Verification items for the finished model (mm, model axes). Face numbers are marked on the shaded views. A direction names the side the tool comes from. Coordinates: 2 decimals unless noted, no trailing zeros. Order: outer loops, then holes, each group sorted by start corner. A loop starts at its lowest first (then second) coordinate and runs counter-clockwise, first axis right, second up. Notation, with made-up numbers: (71, -35) -> (119, -35) arc R27 cw to (119, -14) -> close; hole circle Ø5 at (-28, 37). An arc over 180 degrees is marked (long way). Write item = value, one per line. Start each with the question number.
1. Set-up check for the marked faces 5, 6, 7, 8 and 9: record each of +Z, -Z, +X, -X, +Y, -Y from which the full face is reachable in a straight line by a thin tool's end or side.
2. Release check for a two-part mould opening along X. For the marked faces 1, 2, 3 and 4 record: +X half, -X half, draft (parallel to the pull), parting line (faces both ways), or undercut.
3. Cross-section at A-A on x = -8. Record the cut outline in (y, z), plus the area to 3 significant figures.
4. Cross-section at C-C on x = 0.5. Record the cut outline in (y, z), plus the area to 3 significant figures.
5. Thickness scan on line 1 along Y through (x, z) = (-8, 0.25); line 2 along X through (y, z) = (-26.3, 0); line 3 along Y through (x, z) = (18, 4.5). Record the ranges inside material, lowest first. Write a range as from..to.
6. Go/stop test with flat-tipped pins: P1, Ø1.3, axis at x = 21, z = 0, coming from the +Y side; P2, Ø3, axis at x = 6.5, z = 3, coming from the -Y side; P3, Ø1.5, axis at x = 10, z = -2, coming from the +Y side; P4, Ø4, axis at x = 8, y = -8, coming from the +Z side. Record where each tip stops, or that it passes through.
7. Cross-section at D-D on z = 0. Give the number of separate pieces and of enclosed holes in the cut face, plus the area to 3 significant figures.
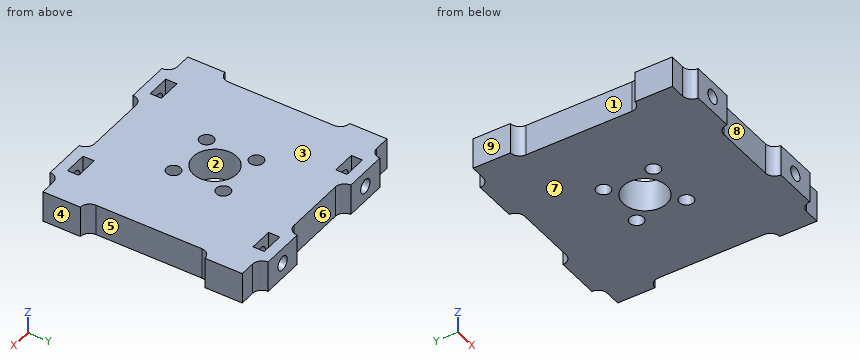
from build123d import *

# Parameters (mm, degrees)
CROQUIS1_W              = 70
CROQUIS1_H              = 70
CROQUIS1_R              = 7
SALIENTE_EXTRUIR1_DEPTH = 5
CROQUIS2_R              = 2.25
CROQUIS2_W              = 26
CROQUIS2_H              = 6
CROQUIS2_W_2            = 6
CROQUIS2_H_2            = 26
CORTAR_EXTRUIR1_DEPTH   = 51.497524692
CROQUIS4_R              = 2.25
CORTAR_EXTRUIR2_DEPTH   = 10
CORTAR_EXTRUIR3_DEPTH   = 3.6
CROQUIS6_W              = 8
CROQUIS6_H              = 3
CROQUIS6_W_2            = 6
CROQUIS6_H_2            = 40
CORTAR_EXTRUIR4_DEPTH   = 51.497524692
REDONDEO1_R             = 3


with BuildPart() as part:
    # Croquis1 → Saliente-Extruir1 (new, symmetric)
    with BuildSketch(Plane.XY):
        Rectangle(CROQUIS1_W, CROQUIS1_H)
        Circle(CROQUIS1_R, mode=Mode.SUBTRACT)
    extrude(amount=SALIENTE_EXTRUIR1_DEPTH, both=True)

    # Croquis2 → Cortar-Extruir1 (cut, through all)
    with BuildSketch(Plane.XY.offset(5)):
        with Locations((8, 8)):
            Circle(CROQUIS2_R)
        with Locations((8, -8)):
            Circle(CROQUIS2_R)
        with Locations((-8, -8)):
            Circle(CROQUIS2_R)
        with Locations((-8, 8)):
            Circle(CROQUIS2_R)
        with Locations((0, 35)):
            Rectangle(CROQUIS2_W, CROQUIS2_H)
        with Locations((-35, 0)):
            Rectangle(CROQUIS2_W_2, CROQUIS2_H_2)
        with Locations((35, 0)):
            Rectangle(CROQUIS2_W_2, CROQUIS2_H_2)
        with Locations((0, -35)):
            Rectangle(CROQUIS2_W, CROQUIS2_H)
    extrude(amount=-CORTAR_EXTRUIR1_DEPTH, mode=Mode.SUBTRACT)

    # Croquis4 → Cortar-Extruir2 (cut)
    with BuildSketch(Plane(origin=(0, 35, 0), x_dir=(1, 0, 0), z_dir=(0, 1, 0))):
        with Locations(Location((-20, 0, 0), (0, 0, 270))):
            Circle(CROQUIS4_R)
        with Locations(Location((20, 0, 0), (0, 0, 270))):
            Circle(CROQUIS4_R)
    cortar_extruir2 = extrude(amount=-CORTAR_EXTRUIR2_DEPTH, mode=Mode.SUBTRACT)

    # Croquis5 → Cortar-Extruir3 (cut)
    with BuildSketch(Plane(origin=(0, 28, 0), x_dir=(1, 0, 0), z_dir=(0, 1, 0))):
        Polygon((-23.75, -2.165063509), (-23.75, -5), (-16.25, -5), (-16.25, -2.165063509), (-16.25, 2.165063509), (-20, 4.330127019), (-23.75, 2.165063509), align=None)
        Polygon((16.25, 2.165063509), (16.25, -2.165063509), (16.25, -5), (23.75, -5), (23.75, -2.165063509), (23.75, 2.165063509), (20, 4.330127019), align=None)
    cortar_extruir3 = extrude(amount=CORTAR_EXTRUIR3_DEPTH, mode=Mode.SUBTRACT)

    # Simetría1: Cortar-Extruir2, Cortar-Extruir3 across plane
    add(cortar_extruir2.mirror(Plane.ZX), mode=Mode.SUBTRACT)
    add(cortar_extruir3.mirror(Plane.ZX), mode=Mode.SUBTRACT)

    # Croquis6 → Cortar-Extruir4 (cut, through all)
    with BuildSketch(Plane.XY.offset(5)):
        with Locations((-31, 33.5)):
            Rectangle(CROQUIS6_W, CROQUIS6_H)
        with Locations((31, 33.5)):
            Rectangle(CROQUIS6_W, CROQUIS6_H)
        with Locations((31, -33.5)):
            Rectangle(CROQUIS6_W, CROQUIS6_H)
        with Locations((-31, -33.5)):
            Rectangle(CROQUIS6_W, CROQUIS6_H)
        with Locations((-35, 0)):
            Rectangle(CROQUIS6_W_2, CROQUIS6_H_2)
        with Locations((35, 0)):
            Rectangle(CROQUIS6_W_2, CROQUIS6_H_2)
    extrude(amount=-CORTAR_EXTRUIR4_DEPTH, mode=Mode.SUBTRACT)

    # Redondeo1
    redondeo1_edges = [part.edges().sort_by_distance(p)[0] for p in [
        (27, -32, 0),
        (13, -32, 0),
        (-13, -32, 0),
        (-27, -32, 0),
        (-32, -20, 0),
        (-32, 20, 0),
        (32, -20, 0),
        (32, 20, 0),
        (27, 32, 0),
        (13, 32, 0),
        (-27, 32, 0),
        (-13, 32, 0),
    ]]
    fillet(redondeo1_edges, radius=REDONDEO1_R - 0.0001)  # a hair under: the kernel refuses the full size


solid = part.part
Worked out:
q1.face_5 = +Z, -Z, +X
q1.face_6 = +Z, -Z, +Y
q1.face_7 = -Z, +X, -X, +Y, -Y
q1.face_8 = +Z, -Z, -Y
q1.face_9 = +Z, -Z, -X, +Y, -Y
q2.face_1 = -X half
q2.face_2 = undercut
q2.face_3 = draft
q2.face_4 = +X half
q3.outline = (-32, -5) -> (-10.25, -5) -> (-10.25, 5) -> (-32, 5) -> close; (-5.75, -5) -> (5.75, -5) -> (5.75, 5) -> (-5.75, 5) -> close; (10.25, -5) -> (32, -5) -> (32, 5) -> (10.25, 5) -> close
q3.area = 550 mm²
q4.outline = (-32, -5) -> (-6.98, -5) -> (-6.98, 5) -> (-32, 5) -> close; (6.98, -5) -> (32, -5) -> (32, 5) -> (6.98, 5) -> close
q4.area = 500 mm²
q5.line_1 = -32..-10.25, -5.75..5.75, 10.25..32
q5.line_2 = -35..-22.25, -17.75..17.75, 22.25..35
q5.line_3 = -35..-31.6, -28..28, 31.6..35
q6.P1 = 25
q6.P2 = -32
q6.P3 = 32.1
q6.P4 = through
q7.separate_pieces = 1
q7.enclosed_holes = 5
q7.area = 3,990 mm²
